Model file for the job. Use its own axes, mm. A direction names the side the tool comes from. Round coordinates to 2 decimals unless told otherwise and drop trailing zeros. Write each loop counter-clockwise with the first axis right and the second up, starting at its lowest first coordinate (ties: lowest second). Pieces come first, ordered by that corner, then holes. Notation, with made-up numbers: (30.25, 63.5) - (66.25, 63.5) arc R15 ccw to (66.25, 78.5) - close; hole circle Ø5 at (42, -4). An arc over 180 degrees is marked (long way). One line per item, written item: value.
from build123d import *

# Parameters (mm, degrees)
SKETCH1_W           = 600
SKETCH1_H           = 450
SKETCH1_W_2         = 549.2
SKETCH1_H_2         = 399.2
BOSS_EXTRUDE1_DEPTH = 25.4
SKETCH2_W           = 25.4
SKETCH2_H           = 25.4
BOSS_EXTRUDE2_DEPTH = 1500
SKETCH3_W           = 600
SKETCH3_H           = 450
SKETCH3_W_2         = 549.2
SKETCH3_H_2         = 399.2
BOSS_EXTRUDE3_DEPTH = 25.4


with BuildPart() as part:
    # Sketch1 → Boss-Extrude1 (new body)
    with BuildSketch(Plane.XY):
        with Locations((300, 225)):
            Rectangle(SKETCH1_W, SKETCH1_H)
        with Locations((300, 225)):
            Rectangle(SKETCH1_W_2, SKETCH1_H_2, mode=Mode.SUBTRACT)
    extrude(amount=BOSS_EXTRUDE1_DEPTH)

    # Sketch2 → Boss-Extrude2 (add)
    with BuildSketch(Plane(origin=(0, 0, 0), x_dir=(-1, 0, 0), z_dir=(0, 0, -1))):
        with Locations((-12.7, 437.3)):
            Rectangle(SKETCH2_W, SKETCH2_H)
        with Locations((-587.3, 437.3)):
            Rectangle(SKETCH2_W, SKETCH2_H)
        with Locations((-587.3, 12.7)):
            Rectangle(SKETCH2_W, SKETCH2_H)
        with Locations((-12.7, 12.7)):
            Rectangle(SKETCH2_W, SKETCH2_H)
    extrude(amount=-BOSS_EXTRUDE2_DEPTH)

    # Sketch3 → Boss-Extrude3 (add)
    with BuildSketch(Plane.XY.offset(1500)):
        with Locations((300, 225)):
            Rectangle(SKETCH3_W, SKETCH3_H)
        with Locations((300, 225)):
            Rectangle(SKETCH3_W_2, SKETCH3_H_2, mode=Mode.SUBTRACT)
    extrude(amount=-BOSS_EXTRUDE3_DEPTH)


solid = part.part
1. Band-saw the part on B-B on y = 335. Write the cut outline in (x, z).
Report:
outline: (0, 0) - (25.4, 0) - (25.4, 25.4) - (0, 25.4) - close; (0, 1474.6) - (25.4, 1474.6) - (25.4, 1500) - (0, 1500) - close; (574.6, 0) - (600, 0) - (600, 25.4) - (574.6, 25.4) - close; (574.6, 1474.6) - (600, 1474.6) - (600, 1500) - (574.6, 1500) - close
2. Mould opens along Z. For faces 6 (the face through (587, 450, 524)), 7 (the face through (296, 13, 1474.6)), 8 (the face through (301, 426, 1500)) say: released by +Z, released by -Z, zero draft, split by the parting line, or undercut.
Report:
face 6: zero draft
face 7: undercut
face 8: released by +Z
3. Tool access for faces 1 (the face through (587, 0, 524)), 2 (the face through (13, 25.4, 740)), 3 (the face through (296, 25.4, 1487)), 4 (the face through (25.4, 13, 740)), 5 (the face through (0, 24, 580)): list every direction of +Z, -Z, +X, -X, +Y, -Y with a clear straight run to the whole face (end or side of a thin tool).
Report:
face 1: +Z, -Z, +X, -X, -Y
face 2: +X, -X
face 3: +Z, -Z
face 4: +Y, -Y
face 5: +Z, -Z, -X, +Y, -Y
4. Band-saw the part on A-A on z = 471. Write the cut outline in (x, y), plus the area to 3 significant figures.
Report:
outline: (0, 0) - (25.4, 0) - (25.4, 25.4) - (0, 25.4) - close; (0, 424.6) - (25.4, 424.6) - (25.4, 450) - (0, 450) - close; (574.6, 0) - (600, 0) - (600, 25.4) - (574.6, 25.4) - close; (574.6, 424.6) - (600, 424.6) - (600, 450) - (574.6, 450) - close
area: 2,580 mm²
5. Drop a flat-ended pin along its axis: pin 1 (20.5 mm diameter, centred on y = 7, z = 645.5, fed in from -X). Give the stop position or say it passes through.
Report:
pin 1: x = 0
